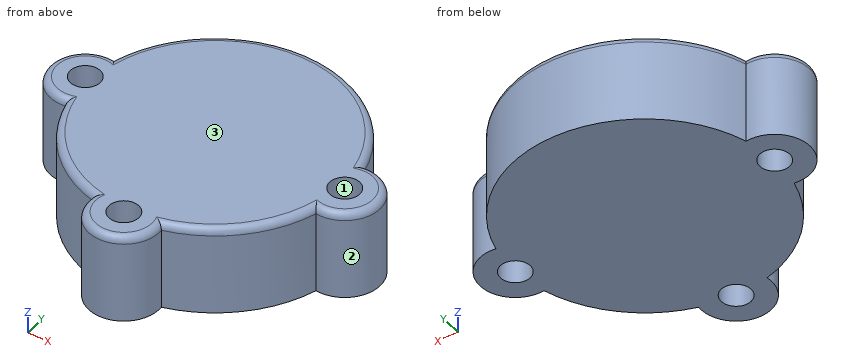
```python
from build123d import *

# Parameters (mm, degrees)
F0_R     = 4.25
F1_DEPTH = 25
F3_R     = 2


# Not quite as in the source:
# - a feature of the source that left no trace in its solid (it failed there, or was rolled back) is left out


with BuildPart() as f1:
    # F0 (on Top) → F1 (new body)
    with BuildSketch(Plane.XY):
        with BuildLine():
            ThreePointArc((36.1666666667, -9.9107124982), (47.5, 0), (36.1666666667, 9.9107124982))
            ThreePointArc((36.1666666667, 9.9107124982), (0, 37.5), (-36.1666666667, 9.9107124982))
            ThreePointArc((-36.1666666667, 9.9107124982), (-47.5, 0), (-36.1666666667, -9.9107124982))
            ThreePointArc((-36.1666666667, -9.9107124982), (-26.5165042945, -26.5165042945), (-9.9107124982, -36.1666666667))
            ThreePointArc((-9.9107124982, -36.1666666667), (0, -47.5), (9.9107124982, -36.1666666667))
            ThreePointArc((9.9107124982, -36.1666666667), (26.5165042945, -26.5165042945), (36.1666666667, -9.9107124982))
        make_face()
        with Locations((0, -37.5)):
            Circle(F0_R, mode=Mode.SUBTRACT)
        with Locations((-37.5, 0)):
            Circle(F0_R, mode=Mode.SUBTRACT)
        with Locations((37.5, 0)):
            Circle(F0_R, mode=Mode.SUBTRACT)
    extrude(amount=F1_DEPTH)

    # F3
    f3_edges = [f1.edges().sort_by_distance(p)[0] for p in [
        (0, -47.5, 25),
        (26.516504, -26.516504, 25),
        (47.5, 0, 25),
        (0, 37.5, 25),
        (-47.5, 0, 25),
        (-26.516504, -26.516504, 25),
    ]]
    fillet(f3_edges, radius=F3_R)


solid = f1.part
```
Verification items for the finished model (mm, model axes). Face numbers are marked on the shaded views. Round coordinates to 2 decimals unless told otherwise and drop trailing zeros. Write each loop counter-clockwise with the first axis right and the second up, starting at its lowest first coordinate (ties: lowest second). Pieces come first, ordered by that corner, then holes.
1. Draft check along Y on the marked faces 1, 2 and 3. Enter one of: +Y half, -Y half, draft (parallel to the pull), parting line (faces both ways), or undercut.
2. Gauge pin test, flat ends, axial feed: P1, Ø4, axis at y = -28, z = 8.5, coming from the +X side; P2, Ø7.5, axis at x = 37.5, y = 0, coming from the +Z side; P3, Ø10, axis at y = 9.5, z = 12.5, coming from the +X side; P4, Ø4, axis at x = 31.5, z = 20.5, coming from the -Y side. Record the tip position at first contact, or that the pin passes through.
3. Section check A-A on x = 0. Enter the section's corners in (y, z), plus the area to 3 significant figures.
4. Section check C-C on z = 17.5. Enter the section's corners in (x, y).
5. Section check B-B on y = 0. Enter the section's corners in (x, z), plus the area to 3 significant figures.
6. Scan lines: L1, parallel to Y at x = 37.5, z = 7.5; L2, parallel to Y at x = 0, z = 7; L3, parallel to X at y = -40, z = 11.5. Record each from-to range of solid material in increasing order.
Answer:
1. face 1: undercut
1. face 2: parting line
1. face 3: draft
2. P1: stops at x = 27.02
2. P2: passes through
2. P3: stops at x = 46.43
2. P4: stops at y = -23.15
3. outline: (-47.5, 0) - (-41.75, 0) - (-41.75, 25) - (-45.5, 25) arc R2 ccw to (-47.5, 23) - close; (-33.25, 0) - (37.5, 0) - (37.5, 23) arc R2 ccw to (35.5, 25) - (-33.25, 25) - close
3. area: 1,910 mm2
4. outline: (-36.17, -9.91) arc R37.5 ccw to (-9.91, -36.17) arc R10 ccw (long way) to (9.91, -36.17) arc R37.5 ccw to (36.17, -9.91) arc R10 ccw (long way) to (36.17, 9.91) arc R37.5 ccw to (-36.17, 9.91) arc R10 ccw (long way) to start; hole circle Ø8.5 at (-37.5, 0); hole circle Ø8.5 at (0, -37.5); hole circle Ø8.5 at (37.5, 0)
5. outline: (-47.5, 0) - (-41.75, 0) - (-41.75, 25) - (-45.5, 25) arc R2 ccw to (-47.5, 23) - close; (-33.25, 0) - (33.25, 0) - (33.25, 25) - (-33.25, 25) - close; (41.75, 0) - (47.5, 0) - (47.5, 23) arc R2 ccw to (45.5, 25) - (41.75, 25) - close
5. area: 1,950 mm2
6. L1: y = -10 to -4.25, 4.25 to 10
6. L2: y = -47.5 to -41.75, -33.25 to 37.5
6. L3: x = -9.68 to -3.44, 3.44 to 9.68
